from build123d import *

# Parameters (mm, degrees)
SKETCH1_R           = 3.175
BOSS_EXTRUDE1_DEPTH = 6.35
FILLET1_R           = 12.7
FILLET2_R           = 3.175


with BuildPart() as part:
    # Sketch1 → Boss-Extrude1 (new body)
    with BuildSketch(Plane(origin=(0, 0, 0), x_dir=(1, 0, 0), z_dir=(0, 1, 0))):
        Polygon((-50.8, 50.8), (-50.8, -50.8), (-76.2, -50.8), (-76.2, -76.2), (-52.3875, -76.2), (-52.3875, -63.5), (52.3875, -63.5), (52.3875, -76.2), (76.2, -76.2), (76.2, -50.8), (50.8, -50.8), (50.8, 50.8), (76.2, 50.8), (76.2, 76.2), (52.3875, 76.2), (52.3875, 63.5), (-52.3875, 63.5), (-52.3875, 76.2), (-76.2, 76.2), (-76.2, 50.8), align=None)
        with Locations(Location((-63.54848247, 63.54848247, 0), (0, 0, 270))):
            Circle(SKETCH1_R, mode=Mode.SUBTRACT)
        with Locations(Location((63.645484454, 63.645484454, 0), (0, 0, 270))):
            Circle(SKETCH1_R, mode=Mode.SUBTRACT)
        with Locations(Location((63.54848247, -63.54848247, 0), (0, 0, 270))):
            Circle(SKETCH1_R, mode=Mode.SUBTRACT)
        with Locations(Location((-63.451480485, -63.451480485, 0), (0, 0, 270))):
            Circle(SKETCH1_R, mode=Mode.SUBTRACT)
    extrude(amount=BOSS_EXTRUDE1_DEPTH)

    # Fillet1
    fillet1_edges = [part.edges().sort_by_distance(p)[0] for p in [
        (50.8, 3.175, -50.8),
        (50.8, 3.175, 50.8),
        (-50.8, 3.175, 50.8),
        (-50.8, 3.175, -50.8),
    ]]
    fillet(fillet1_edges, radius=FILLET1_R)

    # Fillet2
    fillet2_edges = [part.edges().sort_by_distance(p)[0] for p in [
        (-76.2, 3.175, -76.2),
        (-52.3875, 3.175, -76.2),
        (52.3875, 3.175, -76.2),
        (76.2, 3.175, -76.2),
        (76.2, 3.175, -50.8),
        (76.2, 3.175, 50.8),
        (76.2, 3.175, 76.2),
        (52.3875, 3.175, 76.2),
        (-52.3875, 3.175, 76.2),
        (-76.2, 3.175, 76.2),
        (-76.2, 3.175, 50.8),
        (-76.2, 3.175, -50.8),
    ]]
    fillet(fillet2_edges, radius=FILLET2_R)


solid = part.part
Work out the finished part from the listing and answer in its coordinate system (mm). A direction names the side the tool comes from. Give positions to 0.01 mm unless a question says otherwise; leave off trailing zeros. Loops run counter-clockwise (first coordinate to the right, second up) from the corner with the lowest first, then second, coordinate; pieces in that order, holes last. Notation, with made-up numbers: (48, 16) -> (85, 16) arc R14 cw to (85, 28) -> close; hole circle Ø6 at (-31, -0.5). An arc over 180 degrees is marked (long way). Use a Markdown table: item, result. Add a question column.
1. Section C-C on y = 2 is taken. State how many separate pieces and enclosed holes the cut face has, and give its area (3 significant figures).
2. Flat-ended cylindrical pins translate along their axes: pin 1 Ø1.5 at (x, y) = (-4, 4) entering from -Z; pin 2 Ø2 at (y, z) = (0.5, -18) entering from +X; pin 3 Ø1.9 at (x, y) = (17, 4.5) entering from +Z. Find the tip coordinate at first contact, or state that the pin passes through.
3. Section A-A on z = -11 is taken. Determine the outline of the cut face in (x, y), and give its area (3 significant figures).
4. Determine the mould class of faces 1 (the cylindrical face through (-54.42, 3.22, -46.98)), 2 (the cylindrical face through (-54.42, 3.22, 46.98)), 3 (the flat face through (-52.388, 3, -68)), 4 (the flat face through (64, 3, -76.2)) for opening direction Z: released by +Z, released by -Z, zero draft, split by the parting line, or undercut.
5. Find the intervals of material crossed by probe 1 along X at (y, z) = (5, -64); probe 2 along Z at (x, y) = (-68, 0.75); probe 3 along X at (y, z) = (1.25, -67), in increasing order.
6. Section B-B on x = -32 is taken. Determine the outline of the cut face in (y, z).
7. For faces 5 (the flat face through (-1, 3, 63.5)), 6 (the cylindrical face through (54.62, 3.22, 47.18)), 7 (the flat face through (1, 3, -63.5)), 8 (the flat face through (-68, 3, -50.8)), determine the directions among +Z, -Z, +X, -X, +Y, -Y from which every point of the face is accessible in a straight line to the end or side of a thin tool.
Results below:
| question | item | result |
|---|---|---|
| 1 | separate pieces | 1 |
| 1 | enclosed holes | 4 |
| 1 | area | 15,400 mm^2 |
| 2 | pin 1 | stops at z = -63.5 |
| 2 | pin 2 | stops at x = 50.8 |
| 2 | pin 3 | stops at z = 63.5 |
| 3 | outline | (-50.8, 0) -> (50.8, 0) -> (50.8, 6.35) -> (-50.8, 6.35) -> close |
| 3 | area | 645 mm^2 |
| 4 | face 1 | undercut |
| 4 | face 2 | undercut |
| 4 | face 3 | zero draft |
| 4 | face 4 | released by -Z |
| 5 | probe 1 | x = -76.2 to -66.69, -60.41 to -52.39, 52.39 to 60.49, 66.8 to 76.2 |
| 5 | probe 2 | z = -76.2 to -50.8, 50.8 to 76.2 |
| 5 | probe 3 | x = -76.2 to -52.39, 52.39 to 76.2 |
| 6 | outline | (0, -63.5) -> (6.35, -63.5) -> (6.35, 63.5) -> (0, 63.5) -> close |
| 7 | face 5 | +Z, +Y, -Y |
| 7 | face 6 | +X, +Y, -Y |
| 7 | face 7 | -Z, +Y, -Y |
| 7 | face 8 | -X, +Y, -Y |
